Input: part model. Units: mm. Frame: model coordinates. Round coordinates to 2 decimals unless told otherwise and drop trailing zeros. Order: outer loops, then holes, each group sorted by start corner. A loop starts at its lowest first (then second) coordinate and runs counter-clockwise, first axis right, second up. Notation, with made-up numbers: (66.5, 35) -> (124.5, 35) arc R22 ccw to (124.5, 58) -> close; hole circle Ø10 at (-20, -21). An arc over 180 degrees is marked (long way). Answer as CSV lines item,"result". Start each with the question number.
1) Section query A-A, the plane z = 2.5. Output: boundary loops of the cut face in (x, y), and give its area (3 significant figures).
2) First-contact query: P1, Ø10, axis at x = 7.5, y = -5, coming from the +Z side; P2, Ø6, axis at y = 4, z = 5.5, coming from the -X side; P3, Ø4, axis at y = -6.5, z = 4.5, coming from the -X side. Flat tips, straight axial feed; report the tip coordinate or a pass-through.
3) Section query B-B, the plane z = 4. Output: boundary loops of the cut face in (x, y), and give its area (3 significant figures).
4) Line query: L1, parallel to Z at x = 6, y = -3.25; L2, parallel to X at y = -8, z = 7; L3, parallel to Y at x = -6.25, z = 8.25. Output: solid intervals per line, ascending.
5) Mould query, pull axis X, two halves, no side actions, for faces 1 (the face through (2.93, 13.18, 5.22)), 2 (the face through (0, 0, 0)), 3 (the face through (2.553, 11.497, 6.31)). Classes: +X half, -X half, draft (parallel to the pull), parting line (faces both ways), or undercut.
```python
from build123d import *


# Not quite as in the source:
# - a fillet or chamfer that OpenCascade refuses, or shapes differently, is made with other operations: its cross-section is extruded or revolved along the edge and cut away or added


with BuildPart() as f1:
    # F0 (on Front) → F1 (revolve)
    with BuildSketch(Plane.XZ):
        Polygon((-13.5, 0), (0, 0), (0, 2), (-11.65, 2), (-13.5, 2), align=None)
        Polygon((-13.5, 10.5), (-13.5, 2), (-11.65, 2), (-11.9, 10.5), align=None)
    revolve(axis=Axis((0, 0, 1), (0, 0, 1)))

    # F2: fillet of radius 2 on 2 edges, made by hand

    # F2_s1 → F2_t2 (revolve, cut)
    with BuildSketch(Plane.XZ):
        with BuildLine():
            ThreePointArc((-11.9, 10.5), (-13.0491933385, 9.8053192698), (-13.5, 8.5404082058))
            Line((-13.5, 8.5404082058), (-13.5, 10.5))
            Line((-13.5, 10.5), (-11.9, 10.5))
        make_face()
    revolve(axis=Axis((0, 0, 10.5), (0, 0, 1)), mode=Mode.SUBTRACT)

    # F2_s3 → F2_t4 (revolve, cut)
    with BuildSketch(Plane.XZ):
        with BuildLine():
            ThreePointArc((-11.5, 0), (-12.9142135624, 0.5857864376), (-13.5, 2))
            Line((-13.5, 2), (-13.5, 0))
            Line((-13.5, 0), (-11.5, 0))
        make_face()
    revolve(axis=Axis((0, 0, 0), (0, 0, 1)), mode=Mode.SUBTRACT)

    # F3 (on Front) → F4 (revolve, cut)
    with BuildSketch(Plane.XZ):
        with BuildLine():
            Line((11.7787091929, 11.2052995105), (-11.8056663253, 11.404592826))
            ThreePointArc((-11.8056663253, 11.404592826), (-0.1005541056, 1.0004248449), (11.7787091929, 11.2052995105))
        make_face()
    revolve(axis=Axis((-0.0134785662, 0, 11.3049461682), (0.9999642987, 0, -0.0084499248)), mode=Mode.SUBTRACT)


solid = f1.part
```
Findings:
1,outline,"circle Ø27 at (0, 0); hole circle Ø23.33 at (0, 0)"
1,area,"145 mm^2"
2,P1,"stops at z = 10.5"
2,P2,"stops at x = -13.46"
2,P3,"stops at x = -12.73"
3,outline,"circle Ø27 at (0, 0); hole circle Ø23.42 at (0, 0)"
3,area,"142 mm^2"
4,L1,"z = 0 to 2"
4,L2,"x = -10.87 to -8.67, 8.67 to 10.87"
4,L3,"y = -11.97 to -10.05, 10.05 to 11.97"
5,face 1,"parting line"
5,face 2,"draft"
5,face 3,"undercut"
